Read the model definition and answer for the solid it produces. Units are mm, in the model's axes. A direction names the side the tool comes from. Give positions to 0.01 mm unless a question says otherwise; leave off trailing zeros. Write each loop counter-clockwise with the first axis right and the second up, starting at its lowest first coordinate (ties: lowest second). Pieces come first, ordered by that corner, then holes.
```python
from build123d import *

# Parameters (mm, degrees)
BOSS_EXTRUDE1_DEPTH = 3.175
BOSS_EXTRUDE2_DEPTH = 1.27
CUT_EXTRUDE1_DEPTH  = 10.82505851
SCALE1_SCALE        = 2.5


with BuildPart() as part:
    # Sketch2 → Boss-Extrude1 (new, symmetric)
    with BuildSketch(Plane(origin=(0, 0, 0), x_dir=(1, 0, 0), z_dir=(0, 1, 0))):
        with BuildLine():
            Line((-6.274527226, 2.24054867), (-6.274527226, 0.976118894))
            ThreePointArc((-6.274527226, 0.976118894), (0, -1.27), (6.274527226, 0.976118894))
            Line((6.274527226, 0.976118894), (6.274527226, 2.24054867))
            ThreePointArc((6.274527226, 2.24054867), (0, 0), (-6.274527226, 2.24054867))
        make_face()
    extrude(amount=BOSS_EXTRUDE1_DEPTH, both=True)

    # Sketch3 → Boss-Extrude2 (add, symmetric)
    with BuildSketch(Plane(origin=(0, 0, 0), x_dir=(1, 0, 0), z_dir=(0, 1, 0))):
        with BuildLine():
            Line((-4.120326649, -0.370528697), (4.120326649, -0.370528697))
            Line((4.120326649, -0.370528697), (4.120326649, -2.957433704))
            ThreePointArc((4.120326649, -2.957433704), (5.482164962, -4.536659699), (4.120326649, -6.115885694))
            Line((4.120326649, -6.115885694), (-4.120326649, -6.115885694))
            ThreePointArc((-4.120326649, -6.115885694), (-5.482164962, -4.536659699), (-4.120326649, -2.957433704))
            Line((-4.120326649, -2.957433704), (-4.120326649, -0.370528697))
        make_face()
    extrude(amount=BOSS_EXTRUDE2_DEPTH, both=True)

    # Sketch4 → Cut-Extrude1 (cut, through all)
    with BuildSketch(Plane(origin=(0, 1.27, 0), x_dir=(1, 0, 0), z_dir=(0, 1, 0))):
        with BuildLine():
            Line((-3.885588375, -3.966918266), (3.885588375, -3.966918266))
            ThreePointArc((3.885588375, -3.966918266), (4.455329808, -4.536659699), (3.885588375, -5.106401132))
            Line((3.885588375, -5.106401132), (-3.885588375, -5.106401132))
            ThreePointArc((-3.885588375, -5.106401132), (-4.455329808, -4.536659699), (-3.885588375, -3.966918266))
        make_face()
    extrude(amount=-CUT_EXTRUDE1_DEPTH, mode=Mode.SUBTRACT)


with BuildPart() as part_1:
    # Scale1: scaled about (0, 0, 1.671454739)
    add(part.part.scale(SCALE1_SCALE).moved(Location((0, 0, -2.507182109))))


solid = part_1.part
```
Item 1: Section D-D (z = 1) is taken. Write down the section's boundary in (x, y) (3 decimals).
Result set:
outline: (-10.301, -3.175) - (10.301, -3.175) - (10.301, 3.175) - (-10.301, 3.175) - close
Item 2: Each of these flat-tipped pins is pushed along its axis until it touches: pin 1 Ø5 at (y, z) = (3.5, -2) entering from +X; pin 2 Ø5 at (y, z) = (-1.5, 1.5) entering from +X; pin 3 Ø3 at (x, y) = (1.5, 1) entering from -Z; pin 4 Ø3 at (x, z) = (-2.5, -5) entering from +Y. Where does it stop, or does it pass through?
Result set:
pin 1: stops at x = 15.12
pin 2: stops at x = 10.3
pin 3: stops at z = -2.69
pin 4: passes through
Item 3: Section A-A (x = -8.5) is taken. Write down the section's boundary in (y, z) (1 decimal).
Result set:
outline: (-7.9, -4) - (7.9, -4) - (7.9, -0.8) - (3.2, -0.8) - (3.2, 7.4) - (-3.2, 7.4) - (-3.2, -0.8) - (-7.9, -0.8) - close; (-3.2, 10.3) - (3.2, 10.3) - (3.2, 12.8) - (-3.2, 12.8) - close
Item 4: Section B-B (y = 1.5) is taken. Write down the section's boundary in (x, z) (1 decimal), and give its area (3 significant figures).
Result set:
outline: (-15.7, -8.1) arc R24.8 cw to (15.7, -8.1) - (15.7, -4.9) arc R24.7 ccw to (10.3, -1.6) - (10.3, 4.9) arc R4 ccw to (10.3, 12.8) - (-10.3, 12.8) arc R4 ccw to (-10.3, 4.9) - (-10.3, -1.6) arc R24.7 ccw to (-15.7, -4.9) - close; hole (-9.7, 7.4) - (9.7, 7.4) arc R1.4 ccw to (9.7, 10.3) - (-9.7, 10.3) arc R1.4 ccw to start
area: 343 mm2
Item 5: Find the intervals of material crossed by line 1 along X through (y, z) = (-3, -1.25); line 2 along Y through (x, z) = (-11.5, 10.25) (3 decimals); line 3 along X through (y, z) = (-5.25, -4.75), in increasing order.
Result set:
line 1: x = -10.3 to 10.3
line 2: y = -3.175 to 3.175
line 3: x = -15.44 to -10.3, 10.3 to 15.44
Item 6: Which of the six approach directions +Z, -Z, +X, -X, +Y, -Y give full straight-line access (tool end or side, diameter ignored) to faces 1 (the flat face through (0, 0, 10.259)), 2 (the flat face through (-10.301, 0, 2)), 3 (the flat face through (10.301, 0, 2))?
Result set:
face 1: +Y, -Y
face 2: -X, +Y, -Y
face 3: +X, +Y, -Y
Item 7: Section C-C (z = -4) is taken. Write down the section's boundary in (x, y).
Result set:
outline: (-14.46, -7.94) - (-8.47, -7.94) - (-8.47, 7.94) - (-14.46, 7.94) - close; (8.47, -7.94) - (14.46, -7.94) - (14.46, 7.94) - (8.47, 7.94) - close
Item 8: Determine the mould class of faces 4 (the cylindrical face through (-0.238, 3.639, 0.667)), 5 (the cylindrical face through (11.138, 0.044, 8.803)), 6 (the flat face through (15.686, 0, -7)), 7 (the flat face through (-15.686, 0, -7)) for opening direction X: pulls with the +X half, pulls with the -X half, needs draft (parallel to the pull), parting line crosses it, or undercut.
Result set:
face 4: parting line crosses it
face 5: undercut
face 6: pulls with the +X half
face 7: pulls with the -X half
